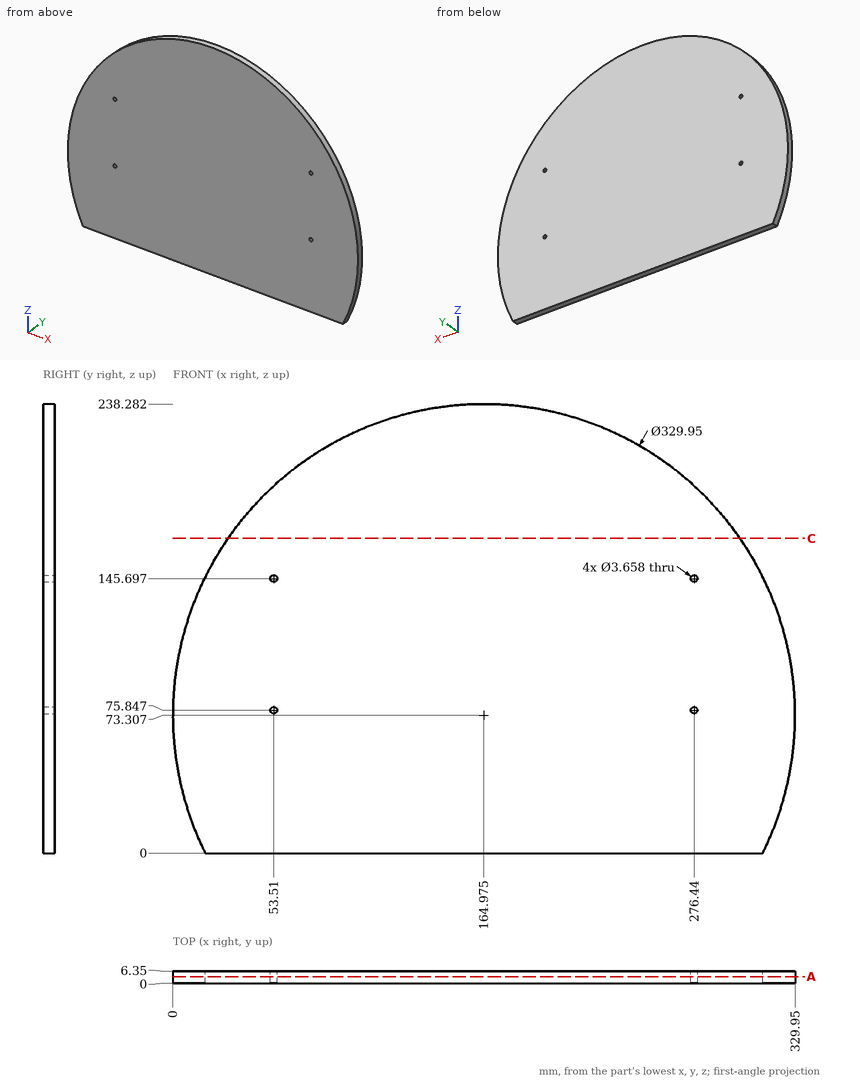
The figure shows three views and two pictorial views of one solid part (mm, origin at its lowest corner). Answer the questions. Coordinates: 2 decimals unless noted, no trailing zeros. Order: outer loops, then holes, each group sorted by start corner. A loop starts at its lowest first (then second) coordinate and runs counter-clockwise, first axis right, second up.
Q1. A cutting plane is placed at A-A, the plane y = 3.5. State how many separate pieces and enclosed holes the cut face has, and give its area (3 significant figures).
Q2. A cutting plane is placed at C-C, the plane z = 167. Write down the section's boundary in (x, y), and give its area (3 significant figures).
Q3. Given P1, Ø2, axis at y = 5.5, z = 158, coming from the +X side (1 decimal); P2, Ø3, axis at y = 3, z = 26, coming from the -X side, each flat-ended and moving along its own axis, determine where each tip first touches the part or whether it passes through.
Q4. Consider line 1 (Z direction, x = 53.51, y = 2.5) (1 decimal); line 2 (X direction, y = 0.75, z = 77); line 3 (Z direction, x = 117.5, y = 2.75) (1 decimal). Determine where each line is inside the solid, lowest interval first.
Answers follow:
1. separate pieces: 1
1. enclosed holes: 4
1. area: 66,100 mm2
2. outline: (29.19, 0) - (300.76, 0) - (300.76, 6.35) - (29.19, 6.35) - close
2. area: 1,720 mm2
3. P1: stops at x = 307.1
3. P2: stops at x = 6.49
4. line 1: z = 0 to 74, 77.7 to 143.9, 147.5 to 194.9
4. line 2: x = 0.04 to 52.09, 54.93 to 275.02, 277.86 to 329.91
4. line 3: z = 0 to 231.3
